Source: three-view drawing plus pictorial views. Frame: mm from the lowest corner of the part. A direction names the side the tool comes from. Give positions to 0.01 mm unless a question says otherwise; leave off trailing zeros. Loops run counter-clockwise (first coordinate to the right, second up) from the corner with the lowest first, then second, coordinate; pieces in that order, holes last. Notation, with made-up numbers: M 26.25,-39 L 47.25,-39 A15 cw 47.25,-23 Z; hole C 75,54 d10. An arc over 180 degrees is marked long. One line per item, written item: value. Start each with the question number.
(1) Access query for the marked faces 1 and 2. Directions: +Z, -Z, +X, -X, +Y, -Y. A direction counts if a zero-diameter tool reaches every point of the face in a straight line with its end or side. Return the directions, or none.
(2) Ray query, line 1 along Y through (x, z) = (28, 16.25) (1 decimal); line 2 along X through (y, z) = (9, 2.75) (1 decimal); line 3 along X through (y, z) = (8, 2) (1 decimal). Return the intervals inside material, ascending. Write a range as from..to.
(3) Pull-direction query (Y, two-part tool) for the marked faces 3, 4 and 5; classes: released by +Y, released by -Y, zero draft, split by the parting line, or undercut.
(4) Section B-B on z = 10. Output: boundary loops of the cut face in (x, y) (1 decimal), plus the area to 3 significant figures.
(5) Section A-A on x = 38. Output: boundary loops of the cut face in (y, z), plus the area to 3 significant figures.
(6) Pin query (flat end, axial travel): P1, Ø1.8, axis at x = 29, y = 22.41, coming from the -Z side; P2, Ø10, axis at x = 56.5, z = 5, coming from the +Y side; P3, Ø4, axis at x = 41.5, z = 9, coming from the -Y side; P4, Ø1.5, axis at y = 58, z = 11.5, coming from the -X side. Return the tip coordinate at first contact, or that it passes through.
(7) Section C-C on z = 2.5. Output: boundary loops of the cut face in (x, y) (1 decimal), plus the area to 3 significant figures.
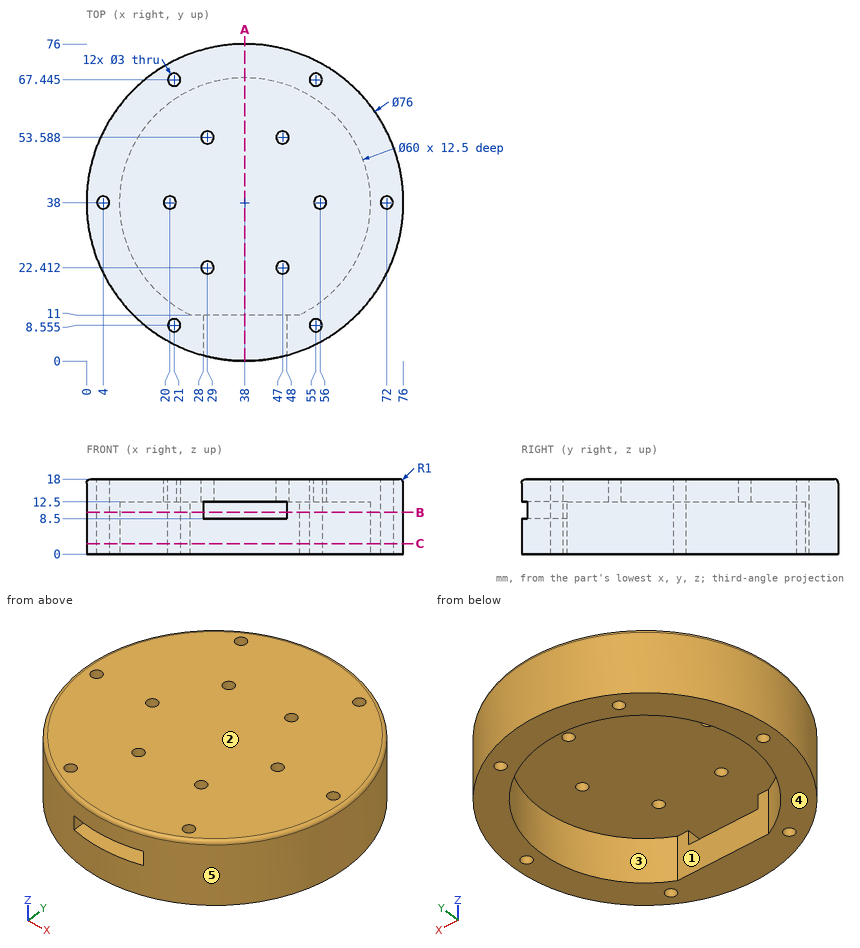
Output values:
1. face 1: -Z
1. face 2: +Z, +X, -X, +Y, -Y
2. line 1: y = 1.3..21.3, 23.5..52.5, 54.7..74.7
2. line 2: x = 13.4..19.6, 22.4..53.6, 56.4..62.6
2. line 3: x = 14.7..19.6, 22.4..53.6, 56.4..61.3
3. face 3: undercut
3. face 4: zero draft
3. face 5: split by the parting line
4. outline: M 24.9,11 A30 cw long 51.1,11 L 48,11 L 48,1.3 A38 ccw long 28,1.3 L 28,11 Z; hole C 4,38 d3; hole C 21,8.6 d3; hole C 21,67.4 d3; hole C 55,8.6 d3; hole C 55,67.4 d3; hole C 72,38 d3
4. area: 1,510 mm²
5. outline: M 0,0 L 11,0 L 11,8.5 L 0,8.5 Z; M 0,12.5 L 68,12.5 L 68,0 L 76,0 L 76,17 A1 ccw 75,18 L 1,18 A1 ccw 0,17 Z
5. area: 611 mm²
6. P1: passes through
6. P2: stops at y = 73.52
6. P3: stops at y = 0.03
6. P4: stops at x = 5.24
7. outline: C 38,38 d76; hole C 4,38 d3; hole C 21,8.6 d3; hole C 21,67.4 d3; hole M 24.9,11 L 51.1,11 A30 ccw long Z; hole C 55,8.6 d3; hole C 55,67.4 d3; hole C 72,38 d3
7. area: 1,720 mm²
